Geometry: final body of the model. Coordinates: model frame, mm. Face numbers are marked on the shaded views. A direction names the side the tool comes from. Give positions to 0.01 mm unless a question says otherwise; leave off trailing zeros. Write each loop counter-clockwise with the first axis right and the second up, starting at its lowest first coordinate (ties: lowest second). Pieces come first, ordered by that corner, then holes. Notation, with made-up numbers: (16, 61.25) - (63, 61.25) arc R19 ccw to (63, 82.25) - close; hole circle Ø8 at (31, -18.5). An arc over 180 degrees is marked (long way). Return JSON: item names as keys, results as strings.
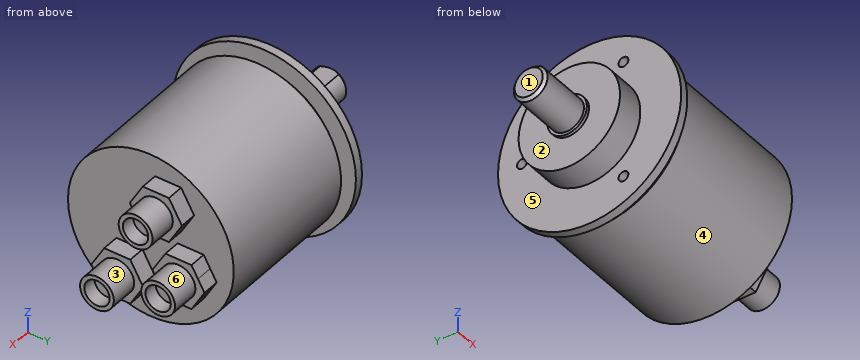
from build123d import *

# Parameters (mm, degrees)
F0_R        = 6
F1_DEPTH    = 18.9
F2_W        = 21.1690347642
F2_H        = 4.931249544
F3_DEPTH    = 18.901
F4_T2_ANGLE = 359.64
F5_R        = 7
F6_DEPTH    = 1.1
F7_R        = 18
F8_DEPTH    = 10
F9_R        = 32.5
F10_DEPTH   = 3
F11_R       = 26
F12_DEPTH   = 3
F14_R       = 29.4
F15_DEPTH   = 52.8
F16_R       = 1.75
F17_DEPTH   = 3
F19_DEPTH   = 6
F20_R       = 6
F21_DEPTH   = 10
F22_R       = 4.5
F23_DEPTH   = 5


# Not quite as in the source:
# - a fillet or chamfer that OpenCascade refuses, or shapes differently, is made with other operations: its cross-section is extruded or revolved along the edge and cut away or added


with BuildPart() as f1:
    # F0 (on Right) → F1 (new body)
    with BuildSketch(Plane.YZ):
        Circle(F0_R)
    extrude(amount=-F1_DEPTH)

    # F2 (on Right) → F3 (cut, through all)
    with BuildSketch(Plane.YZ):
        with Locations((0.0764410943, 7.465624772)):
            Rectangle(F2_W, F2_H)
    extrude(amount=-F3_DEPTH, mode=Mode.SUBTRACT)

    # F4: chamfer of 1 on 1 edges, made by hand

    # F4_s1 → F4_t2 (revolve, cut)
    with BuildSketch(Plane(origin=(0, 0, 0), x_dir=(1, 0, 0), z_dir=(0, 0.9999950652, 0.0031415875))):
        with BuildLine():
            Line((-17.8717157288, -6.0282842712), (-18.9282842712, -4.9717157288))
            Line((-18.9282842712, -4.9717157288), (-18.9482842712, -4.9717157288))
            ThreePointArc((-18.9482842712, -4.9717157288), (-18.92, -5.4858578644), (-18.92, -6))
            Line((-18.92, -6), (-18.9, -6.02))
            ThreePointArc((-18.9, -6.02), (-18.3858578644, -6.02), (-17.8717157288, -6.0482842712))
            Line((-17.8717157288, -6.0482842712), (-17.8717157288, -6.0282842712))
        make_face()
    revolve(axis=Axis((-18.9, 0, 0), (1, 0, 0)), revolution_arc=F4_T2_ANGLE, mode=Mode.SUBTRACT)

    # F5 (on face) → F6 (join)
    with BuildSketch(Plane.YZ):
        Circle(F5_R)
    extrude(amount=F6_DEPTH)

    # F7 (on face) → F8 (join)
    with BuildSketch(Plane.YZ.offset(1.1)):
        Circle(F7_R)
    extrude(amount=F8_DEPTH)

    # F9 (on face) → F10 (join)
    with BuildSketch(Plane.YZ.offset(11.1)):
        Circle(F9_R)
    extrude(amount=F10_DEPTH)

    # F11 (on face) → F12 (join)
    with BuildSketch(Plane.YZ.offset(14.1)):
        Circle(F11_R)
    extrude(amount=F12_DEPTH)

    # F14 (on offset) → F15 (join, through all)
    with BuildSketch(Plane(origin=(69.9, 0, 0), x_dir=(0, -1, 0), z_dir=(-1, 0, 0))):
        Circle(F14_R)
    extrude(amount=F15_DEPTH)

    # F16 (on face) → F17 (cut)
    with BuildSketch(Plane(origin=(11.1, 0, 0), x_dir=(0, -1, 0), z_dir=(-1, 0, 0))):
        with Locations((-24, 0)):
            Circle(F16_R)
        with Locations((12, -20.7846096908)):
            Circle(F16_R)
        with Locations((12, 20.7846096908)):
            Circle(F16_R)
    extrude(amount=-F17_DEPTH, mode=Mode.SUBTRACT)

    # F18 (on face) → F19 (join)
    with BuildSketch(Plane.YZ.offset(69.9)):
        with BuildLine():
            ThreePointArc((21.0282031968, -10.574938038), (21.8274066017, -8.6454903731), (22.1, -6.57493798))
            ThreePointArc((22.1, -6.57493798), (21.8274066078, -4.5043856099), (21.0282032207, -2.5749379634))
            ThreePointArc((21.0282032207, -2.5749379634), (18.0999999917, 0.3532652551), (14.1, 1.42506202))
            ThreePointArc((14.1, 1.42506202), (10.1000001451, 0.3532653341), (7.1717969373, -2.5749376897))
            ThreePointArc((7.1717969373, -2.5749376897), (6.1, -6.5749379695), (7.1717969269, -10.5749382522))
            ThreePointArc((7.1717969269, -10.5749382522), (10.1000001361, -13.5031412888), (14.1, -14.57493798))
            ThreePointArc((14.1, -14.57493798), (18.099999971, -13.503141227), (21.0282031968, -10.574938038))
        make_face()
        with BuildLine():
            ThreePointArc((21.0282032207, -2.5749379634), (21.8274066078, -4.5043856099), (22.1, -6.57493798))
            ThreePointArc((22.1, -6.57493798), (21.8274066017, -8.6454903731), (21.0282031968, -10.574938038))
            Line((21.0282031968, -10.574938038), (23.337604307, -6.57493798))
            Line((23.337604307, -6.57493798), (21.0282032207, -2.5749379634))
        make_face()
        with BuildLine():
            ThreePointArc((14.1, 1.42506202), (18.0999999917, 0.3532652551), (21.0282032207, -2.5749379634))
            Line((21.0282032207, -2.5749379634), (18.7188021535, 1.42506202))
            Line((18.7188021535, 1.42506202), (14.1, 1.42506202))
        make_face()
        with BuildLine():
            Line((18.7188021535, -14.57493798), (21.0282031968, -10.574938038))
            ThreePointArc((21.0282031968, -10.574938038), (18.099999971, -13.503141227), (14.1, -14.57493798))
            Line((14.1, -14.57493798), (18.7188021535, -14.57493798))
        make_face()
        with BuildLine():
            ThreePointArc((7.1717969373, -2.5749376897), (10.1000001451, 0.3532653341), (14.1, 1.42506202))
            Line((14.1, 1.42506202), (9.4811978465, 1.42506202))
            Line((9.4811978465, 1.42506202), (7.1717969373, -2.5749376897))
        make_face()
        with BuildLine():
            Line((9.4811978465, -14.57493798), (14.1, -14.57493798))
            ThreePointArc((14.1, -14.57493798), (10.1000001361, -13.5031412888), (7.1717969269, -10.5749382522))
            Line((7.1717969269, -10.5749382522), (9.4811978465, -14.57493798))
        make_face()
        with BuildLine():
            ThreePointArc((7.1717969269, -10.5749382522), (6.1, -6.5749379695), (7.1717969373, -2.5749376897))
            Line((7.1717969373, -2.5749376897), (4.862395693, -6.57493798))
            Line((4.862395693, -6.57493798), (7.1717969269, -10.5749382522))
        make_face()
        Polygon((10.7188021535, 22.2), (1.4811978465, 22.2), (-3.137604307, 14.2), (1.4811978465, 6.2), (10.7188021535, 6.2), (15.337604307, 14.2), align=None)
        Polygon((-2.9811978465, -6.4), (-12.2188021535, -6.4), (-16.837604307, -14.4), (-12.2188021535, -22.4), (-2.9811978465, -22.4), (1.637604307, -14.4), align=None)
    extrude(amount=F19_DEPTH)

    # F20 (on face) → F21 (join)
    with BuildSketch(Plane.YZ.offset(75.9)):
        with Locations((6.1, 14.2)):
            Circle(F20_R)
        with Locations((14.1, -6.57493798)):
            Circle(F20_R)
        with Locations((-7.6, -14.4)):
            Circle(F20_R)
    extrude(amount=F21_DEPTH)

    # F22 (on face) → F23 (cut)
    with BuildSketch(Plane.YZ.offset(85.9)):
        with Locations((6.1, 14.2)):
            Circle(F22_R)
        with Locations((-7.6, -14.4)):
            Circle(F22_R)
        with Locations((14.1, -6.57493798)):
            Circle(F22_R)
    extrude(amount=-F23_DEPTH, mode=Mode.SUBTRACT)


solid = f1.part
Q1. Material intervals for probe 1 along X at (y, z) = (-19, -19); probe 2 along Z at (x, y) = (84, -7.6); probe 3 along Z at (x, y) = (84.7, 14.1), sorted ascending. Write a range as [from, to].
Answer key:
{"probe 1": "x = [11.1, 14.1], [17.1, 69.9]", "probe 2": "z = [-20.4, -18.9], [-9.9, -8.4]", "probe 3": "z = [-12.57, -11.07], [-2.07, -0.57]"}
Q2. Section query C-C, the plane z = 16. Return the cut outline in (x, y).
Answer key:
{"outline": "(1.1, -8.25) - (11.1, -8.25) - (11.1, -28.29) - (14.1, -28.29) - (14.1, -20.49) - (17.1, -20.49) - (17.1, -24.66) - (69.9, -24.66) - (69.9, -2.1) - (75.9, -2.1) - (75.9, 0.38) - (85.9, 0.38) - (85.9, 1.98) - (80.9, 1.98) - (80.9, 10.22) - (85.9, 10.22) - (85.9, 11.82) - (75.9, 11.82) - (75.9, 14.3) - (69.9, 14.3) - (69.9, 24.66) - (17.1, 24.66) - (17.1, 20.49) - (14.1, 20.49) - (14.1, 28.29) - (11.1, 28.29) - (11.1, 8.25) - (1.1, 8.25) - close"}
Q3. Section query A-A, the plane z = -28. Return the cut outline in (x, y).
Answer key:
{"outline": "(11.1, -16.5) - (14.1, -16.5) - (14.1, 16.5) - (11.1, 16.5) - close; (17.1, -8.96) - (69.9, -8.96) - (69.9, 8.96) - (17.1, 8.96) - close"}
Q4. Section query B-B, the plane x = 26. Return the cut outline in (y, z), plus the area to 3 significant figures.
Answer key:
{"outline": "circle Ø58.8 at (0, 0)", "area": "2,720 mm^2"}
Q5. Mould query, pull axis Y, two halves, no side actions, for the marked faces 4, 5 and 6. Classes: pulls with the +Y half, pulls with the -Y half, needs draft (parallel to the pull), parting line crosses it, or undercut.
Answer key:
{"face 4": "parting line crosses it", "face 5": "needs draft", "face 6": "undercut"}
Q6. Pin query (flat end, axial travel): P1, Ø2, axis at x = 24.5, z = 1, coming from the +Y side; P2, Ø4.5, axis at y = -7, z = -12.5, coming from the +X side; P3, Ø10, axis at x = 22, y = 2.5, coming from the +Z side; P4, Ø4.5, axis at y = 12, z = -5.5, coming from the +X side. Return the tip coordinate at first contact, or that it passes through.
Answer key:
{"P1": "stops at y = 29.4", "P2": "stops at x = 80.9", "P3": "stops at z = 29.4", "P4": "stops at x = 85.9"}
Q7. Set-up query: the marked faces 1, 2 and 3. Return all of +Z, -Z, +X, -X, +Y, -Y with unobstructed straight access to the full face (end or side cutting, diameter ignored); none if empty.
Answer key:
{"face 1": "+Z, -Z, -X, +Y, -Y", "face 2": "-X", "face 3": "+X"}
